Geometry check sheet. Reference: the model listing, model coordinates, mm. A direction names the side the tool comes from. Coordinates: 2 decimals unless noted, no trailing zeros. Loops run counter-clockwise (first coordinate to the right, second up) from the corner with the lowest first, then second, coordinate; pieces in that order, holes last. Notation, with made-up numbers: (22, 85.5) - (45, 85.5) arc R21 ccw to (45, 111.5) - close; hole circle Ø6 at (71, 61). An arc over 180 degrees is marked (long way). Write item = value, one per line. Start each with the question number.
from build123d import *

# Parameters (mm, degrees)
SKETCH_1_R          = 3
SKETCH_1_R_2        = 2
EXTRUDE_1_DEPTH     = 7
SKETCH_2_R          = 2
EXTRUDE_2_DEPTH     = 7
CHAMFER_1_SIZE      = 0.5
CHAMFER_1_SIZE2     = 0.365244226
SKETCH_3_W          = 2
SKETCH_3_H          = 0.5
CUT_EXTRUDE_1_DEPTH = 7
SKETCH_4_W          = 2
SKETCH_4_H          = 7
EXTRUDE_3_DEPTH     = 0.5


with BuildPart() as part:
    # 草图1 → 凸台-拉伸1 (new body)
    with BuildSketch(Plane.XY):
        Circle(SKETCH_1_R)
        Circle(SKETCH_1_R_2, mode=Mode.SUBTRACT)
    extrude(amount=EXTRUDE_1_DEPTH)

    # 草图2 → 凸台-拉伸2 (add)
    with BuildSketch(Plane(origin=(0, 0, 0), x_dir=(-1, 0, 0), z_dir=(0, 0, -1))):
        with BuildLine():
            Line((0.378213472, 2.976063603), (15.378213472, 2.976063603))
            Line((15.378213472, 2.976063603), (23.378213472, -1.64273855))
            Line((23.378213472, -1.64273855), (28.699571557, -9.91799539))
            Line((28.699571557, -9.91799539), (15, -3))
            Line((15, -3), (0, -3))
            ThreePointArc((0, -3), (-2.994009921, 0.189485079), (0.378213472, 2.976063603))
        make_face()
        with Locations(Location((0, 0, 0), (0, 0, 180))):
            Circle(SKETCH_2_R, mode=Mode.SUBTRACT)
    extrude(amount=-EXTRUDE_2_DEPTH)

    # 倒角1
    chamfer_1_edges = [part.edges().sort_by_distance(p)[0] for p in [
        (-28.699571557, -9.91799539, 3.5),
    ]]
    chamfer_1_side = [part.faces().sort_by_distance(p)[0] for p in [
        (-26.038892515, -5.78036697, 3.5),
    ]]
    chamfer(chamfer_1_edges, length=CHAMFER_1_SIZE, length2=CHAMFER_1_SIZE2, reference=chamfer_1_side[0])

    # 草图3 → 切除-拉伸1 (cut)
    with BuildSketch(Plane(origin=(0, 0, 0), x_dir=(-1, 0, 0), z_dir=(0, 0, -1))):
        with Locations((11, 2.726063603)):
            Rectangle(SKETCH_3_W, SKETCH_3_H)
        Polygon((17.002138833, 2.038489859), (16.752138833, 1.605477157), (18.484189641, 0.605477157), (18.734189641, 1.038489859), align=None)
    extrude(amount=-CUT_EXTRUDE_1_DEPTH, mode=Mode.SUBTRACT)

    # 草图4 → 凸台-拉伸3 (add)
    with BuildSketch(Plane(origin=(0, 2.476063603, 0), x_dir=(1, 0, 0), z_dir=(0, 1, 0))):
        with Locations((-11, -3.5)):
            Rectangle(SKETCH_4_W, SKETCH_4_H)
    extrude(amount=EXTRUDE_3_DEPTH)


solid = part.part
(1) Tool access check on faces 1 (the face through (-8, -3, 3)), 2 (the face through (-13, -1, 7)). Record the directions out of +Z, -Z, +X, -X, +Y, -Y that give a thin tool (end or side, any length) a straight path to the whole face; none if there is none.
(2) Sectioned sample at B-B on y = 0. Enter the section's corners in (x, z).
(3) Sectioned sample at C-C on x = -7.5. Enter the section's corners in (y, z), plus the area to 3 significant figures.
(4) Sectioned sample at A-A on z = 2.5. Enter the section's corners in (x, y), plus the area to 3 significant figures.
(5) Depth check by flat-ended pin: pin 1 (1.5 mm diameter, centred on y = -1, z = 5.5, fed in from +X); pin 2 (4 mm diameter, centred on x = -1.5, z = 3, fed in from -Y); pin 3 (3 mm diameter, centred on y = -0.5, z = 5, fed in from -X). Enter the tip coordinate at first touch or a pass-through.
(6) Scan lines: line 1 (Y direction, x = 0, z = 1); line 2 (Y direction, x = -10, z = 1.75); line 3 (X direction, y = 1.75, z = 5.25). Record each from-to range of solid material in increasing order.
(7) Sectioned sample at D-D on y = -2.5. Enter the section's corners in (x, z), plus the area to 3 significant figures.
(8) Draft check along X on faces 3 (the face through (-8, 2.976, 3)), 4 (the face through (-16.2, 2.5, 3.5)), 5 (the face through (-17.61, 1.11, 3.45)), 6 (the face through (-21.78, -6.424, 3.451)). Enter one of: pulls with the +X half, pulls with the -X half, needs draft (parallel to the pull), parting line crosses it, or undercut.
Working result:
q1.face_1 = +Z, -Z, +X, -Y
q1.face_2 = +Z, +X, -X, +Y, -Y
q2.outline = (-20.53, 0) - (-2, 0) - (-2, 7) - (-20.53, 7) - close; (2, 0) - (3, 0) - (3, 7) - (2, 7) - close
q3.outline = (-3, 0) - (2.98, 0) - (2.98, 7) - (-3, 7) - close
q3.area = 41.8 mm2
q4.outline = (-28.43, -9.5) - (-28.37, -9.75) - (-15, -3) - (0, -3) arc R3 ccw (long way) to (-0.38, 2.98) - (-15.38, 2.98) - (-17, 2.04) - (-16.75, 1.61) - (-18.48, 0.61) - (-18.73, 1.04) - (-23.38, -1.64) - close; hole circle Ø4 at (0, 0)
q4.area = 154 mm2
q5.pin_1 = 2.99
q5.pin_2 = -3
q5.pin_3 = -23.61
q6.line_1 = -3 to -2, 2 to 3
q6.line_2 = -3 to 2.98
q6.line_3 = -16.84 to -0.97, 0.97 to 2.44
q7.outline = (-23.93, 0) - (1.66, 0) - (1.66, 7) - (-23.93, 7) - close
q7.area = 179 mm2
q8.face_3 = needs draft
q8.face_4 = pulls with the -X half
q8.face_5 = undercut
q8.face_6 = pulls with the +X half
